Part model, mm, in its own coordinate system. A direction names the side the tool comes from. Round coordinates to 2 decimals unless told otherwise and drop trailing zeros. Loops run counter-clockwise (first coordinate to the right, second up) from the corner with the lowest first, then second, coordinate; pieces in that order, holes last.
from build123d import *

# Parameters (mm, degrees)
SKETCH3_R           = 0.635
BOSS_EXTRUDE2_DEPTH = 2.54
SKETCH4_W           = 165.279862668
SKETCH4_H           = 127
CUT_EXTRUDE1_DEPTH  = 125.579462115
FILLET3_R           = 6.35


with BuildPart() as part:
    # Sketch3 → Boss-Extrude2 (new body)
    with BuildSketch(Plane(origin=(0, 0, 0), x_dir=(1, 0, 0), z_dir=(0, 1, 0))):
        Polygon((-75.438, 48.30953), (-75.438, -99.10953), (-47.752, -99.10953), (-47.752, 3.51009118), (-47.752, 43.22953), (47.752, 43.22953), (47.752, 3.51009118), (47.752, -99.10953), (75.438, -99.10953), (75.438, 48.30953), (75.438, 70.50296882), (25.4, 70.50296882), (25.4, 99.10953), (-25.4, 99.10953), (-25.4, 70.50296882), (-75.438, 70.50296882), align=None)
        with Locations(Location((-61.595, 43.22953, 0), (0, 0, 270))):
            Circle(SKETCH3_R, mode=Mode.SUBTRACT)
        with Locations(Location((-70.358, 34.46653, 0), (0, 0, 270))):
            Circle(SKETCH3_R, mode=Mode.SUBTRACT)
        with Locations(Location((-61.595, 25.70353, 0), (0, 0, 270))):
            Circle(SKETCH3_R, mode=Mode.SUBTRACT)
        with Locations(Location((-52.832, 34.46653, 0), (0, 0, 270))):
            Circle(SKETCH3_R, mode=Mode.SUBTRACT)
        with Locations(Location((-52.832, -34.46653, 0), (0, 0, 90))):
            Circle(SKETCH3_R, mode=Mode.SUBTRACT)
        with Locations(Location((-61.595, -25.70353, 0), (0, 0, 90))):
            Circle(SKETCH3_R, mode=Mode.SUBTRACT)
        with Locations(Location((-70.358, -34.46653, 0), (0, 0, 90))):
            Circle(SKETCH3_R, mode=Mode.SUBTRACT)
        with Locations(Location((-61.595, -43.22953, 0), (0, 0, 90))):
            Circle(SKETCH3_R, mode=Mode.SUBTRACT)
        with Locations(Location((61.595, -43.22953, 0), (0, 0, 270))):
            Circle(SKETCH3_R, mode=Mode.SUBTRACT)
        with Locations(Location((61.595, -25.70353, 0), (0, 0, 270))):
            Circle(SKETCH3_R, mode=Mode.SUBTRACT)
        with Locations(Location((52.832, -34.46653, 0), (0, 0, 270))):
            Circle(SKETCH3_R, mode=Mode.SUBTRACT)
        with Locations(Location((52.832, 34.46653, 0), (0, 0, 90))):
            Circle(SKETCH3_R, mode=Mode.SUBTRACT)
        with Locations(Location((61.595, 25.70353, 0), (0, 0, 90))):
            Circle(SKETCH3_R, mode=Mode.SUBTRACT)
        with Locations(Location((61.595, 43.22953, 0), (0, 0, 90))):
            Circle(SKETCH3_R, mode=Mode.SUBTRACT)
        with Locations(Location((70.358, -34.46653, 0), (0, 0, 270))):
            Circle(SKETCH3_R, mode=Mode.SUBTRACT)
        with Locations(Location((70.358, 34.46653, 0), (0, 0, 270))):
            Circle(SKETCH3_R, mode=Mode.SUBTRACT)
    extrude(amount=BOSS_EXTRUDE2_DEPTH)

    # Sketch4 → Cut-Extrude1 (cut, through all)
    with BuildSketch(Plane(origin=(0, 2.54, 0), x_dir=(1, 0, 0), z_dir=(0, 1, 0))):
        with Locations((3.512659274, -111.80953)):
            Rectangle(SKETCH4_W, SKETCH4_H)
    extrude(amount=-CUT_EXTRUDE1_DEPTH, mode=Mode.SUBTRACT)

    # Fillet3
    fillet3_edges = [part.edges().sort_by_distance(p)[0] for p in [
        (75.438, 1.27, 48.30953),
        (-75.438, 1.27, 48.30953),
        (-47.752, 1.27, 48.30953),
        (47.752, 1.27, 48.30953),
        (-75.438, 1.27, -70.50296882),
        (-25.4, 1.27, -70.50296882),
        (-25.4, 1.27, -99.10953),
        (25.4, 1.27, -99.10953),
        (25.4, 1.27, -70.50296882),
        (75.438, 1.27, -70.50296882),
        (47.752, 1.27, -43.22953),
        (-47.752, 1.27, -43.22953),
    ]]
    fillet(fillet3_edges, radius=FILLET3_R)


solid = part.part
1) Slice it at B-B, the plane x = 7. Give the cut face in (y, z).
Values:
outline: (0, -99.11) - (2.54, -99.11) - (2.54, -43.23) - (0, -43.23) - close
2) Slice it at D-D, the plane z = -79.5. Give the cut face in (x, y).
Values:
outline: (-25.4, 0) - (25.4, 0) - (25.4, 2.54) - (-25.4, 2.54) - close
3) Mould opens along X. For faces 1 (the face through (49.66, 1.25, 46.5)), 2 (the face through (-23.59, 1.29, -97.2)), 3 (the face through (23.49, 1.29, -97.3)), 4 (the face through (45.94, 1.29, -41.32)) say: released by +X, released by -X, zero draft, split by the parting line, or undercut.
Values:
face 1: undercut
face 2: released by -X
face 3: released by +X
face 4: undercut
4) Slice it at A-A, the plane z = -29. Give the cut face in (x, y), then the cut area to 3 significant figures.
Values:
outline: (-75.44, 0) - (-47.75, 0) - (-47.75, 2.54) - (-75.44, 2.54) - close; (47.75, 0) - (75.44, 0) - (75.44, 2.54) - (47.75, 2.54) - close
area: 141 mm2
5) Tool access for faces 5 (the face through (-45.84, 1.29, -41.42)), 6 (the face through (27.211, 1.288, -72.412)): list every direction of +Z, -Z, +X, -X, +Y, -Y with a clear straight run to the whole face (end or side of a thin tool).
Values:
face 5: +Z, +Y, -Y
face 6: -Z, +X, +Y, -Y
6) Slice it at C-C, the plane y = 0.55. Give the number of separate pieces and of enclosed holes in the cut face, then the cut area to 3 significant figures.
Values:
separate pieces: 1
enclosed holes: 16
area: 10,600 mm2
7) Drop a flat-ended pin along its axis: pin 1 Ø1.5 at (x, y) = (-13, 1) entering from +Z. Give the stop position or say it passes through.
Values:
pin 1: stops at z = -43.23
8) Wall check: line 1 along X through (y, z) = (1.9, 12); line 2 along X through (y, z) = (2, -80); line 3 along Z through (x, y) = (55.5, 0.65). Give the ranges that are in metal, low to high.
Values:
line 1: x = -75.44 to -47.75, 47.75 to 75.44
line 2: x = -25.4 to 25.4
line 3: z = -70.5 to 48.31
